from build123d import *

# Parameters (mm, degrees)
F0_R     = 11
F1_DEPTH = 7


# Not quite as in the source:
# - a feature of the source that left no trace in its solid (it failed there, or was rolled back) is left out


with BuildPart() as f1:
    # F0 (on Top) → F1 (new body)
    with BuildSketch(Plane.XY):
        with BuildLine():
            ThreePointArc((10.0491768514, 24.5005127008), (2.4404784534, 18.2483589799), (-7.1242678109, 20.5930010332))
            ThreePointArc((-7.1242678109, 20.5930010332), (-12.6262898219, 5.3096518199), (-26.2426548303, -3.54741391))
            ThreePointArc((-26.2426548303, -3.54741391), (-17.732134245, -6.3123707797), (-14.0924093757, -14.4871093077))
            ThreePointArc((-14.0924093757, -14.4871093077), (-14.1373809935, -15.4807657603), (-14.2719281295, -16.4662974242))
            ThreePointArc((-14.2719281295, -16.4662974242), (1.7148515496, -13.5895136513), (16.1934779789, -20.9530987908))
            ThreePointArc((16.1934779789, -20.9530987908), (14.5833032273, -11.237695828), (21.3961959404, -4.126703609))
            ThreePointArc((21.3961959404, -4.126703609), (10.9114382722, 8.2798618313), (10.0491768514, 24.5005127008))
        make_face()
        Circle(F0_R, mode=Mode.SUBTRACT)
        with BuildLine():
            ThreePointArc((10.0491768514, 24.5005127008), (10.7596687999, 26.6874026373), (11, 28.9742186153))
            ThreePointArc((11, 28.9742186153), (-4.6169824604, 38.9583797198), (-7.1242678109, 20.5930010332))
            ThreePointArc((-7.1242678109, 20.5930010332), (2.4404784534, 18.2483589799), (10.0491768514, 24.5005127008))
        make_face()
        with BuildLine():
            ThreePointArc((-14.0924093757, -14.4871093077), (-17.732134245, -6.3123707797), (-26.2426548303, -3.54741391))
            ThreePointArc((-26.2426548303, -3.54741391), (-33.1610370706, -21.9635554634), (-14.2719281295, -16.4662974242))
            ThreePointArc((-14.2719281295, -16.4662974242), (-14.1373809935, -15.4807657603), (-14.0924093757, -14.4871093077))
        make_face()
        with BuildLine():
            ThreePointArc((36.0924093757, -14.4871093077), (31.4304552974, -5.4966046559), (21.3961959404, -4.126703609))
            ThreePointArc((21.3961959404, -4.126703609), (14.5833032273, -11.237695828), (16.1934779789, -20.9530987908))
            ThreePointArc((16.1934779789, -20.9530987908), (28.4918030448, -24.9486638137), (36.0924093757, -14.4871093077))
        make_face()
    extrude(amount=F1_DEPTH)


solid = f1.part
Geometry check sheet. Reference: the model listing, model coordinates, mm. Coordinates: 2 decimals unless noted, no trailing zeros. Order: outer loops, then holes, each group sorted by start corner. A loop starts at its lowest first (then second) coordinate and runs counter-clockwise, first axis right, second up. Notation, with made-up numbers: (27, 20) -> (47, 20) arc R22 ccw to (47, 26) -> close; hole circle Ø5 at (-40, 3). An arc over 180 degrees is marked (long way). Use a Markdown table: item, result. Add a question column.
1. Cross-section at A-A (y = -18). Enter the section's corners in (x, z), and give its area (3 significant figures).
2. Cross-section at B-B (z = 2.75). Enter the section's corners in (x, y), and give its area (3 significant figures).
3. Go/stop test with flat-tipped pins: pin 1 Ø3 at (x, z) = (18, 5) entering from -Y; pin 2 Ø1 at (y, z) = (1, 3.5) entering from +X; pin 3 Ø2 at (y, z) = (-12.5, 5.5) entering from -X. Record where each tip stops, or that it passes through.
4. Cross-section at D-D (x = -27.5). Enter the section's corners in (y, z).
5. Mould release check, pull along Y, two halves, no side actions. Record for faces 1 (the face through (-9, 8, 0)), 2 (the face through (-12.483, 5.492, 3.451)), 3 (the face through (1.486, -13.557, 3.451)): pulls with the +Y half, pulls with the -Y half, needs draft (parallel to the pull), parting line crosses it, or undercut.
6. Cross-section at C-C (x = 0). Enter the section's corners in (y, z).
7. Material ranges on L1, parallel to Y at x = -0.5, z = 1; L2, parallel to Y at x = 6, z = 4.75; L3, parallel to Y at x = 28, z = 0.5, recorded low to high.
Filled sheet:
| question | item | result |
|---|---|---|
| 1 | outline | (-35.52, 0) -> (-14.67, 0) -> (-14.67, 7) -> (-35.52, 7) -> close; (12.72, 0) -> (35.52, 0) -> (35.52, 7) -> (12.72, 7) -> close |
| 1 | area | 305 mm2 |
| 2 | outline | (-26.24, -3.55) arc R11 ccw (long way) to (-14.27, -16.47) arc R25.49 cw to (16.19, -20.95) arc R11 ccw (long way) to (21.4, -4.13) arc R25.49 cw to (10.05, 24.5) arc R11 ccw (long way) to (-7.12, 20.59) arc R25.49 cw to start; hole circle Ø22 at (0, 0) |
| 2 | area | 1,690 mm2 |
| 3 | pin 1 | y = -23.96 |
| 3 | pin 2 | x = 15.77 |
| 3 | pin 3 | x = -36.05 |
| 4 | outline | (-25.22, 0) -> (-3.75, 0) -> (-3.75, 7) -> (-25.22, 7) -> close |
| 5 | face 1 | needs draft |
| 5 | face 2 | undercut |
| 5 | face 3 | pulls with the -Y half |
| 6 | outline | (-13.4, 0) -> (-11, 0) -> (-11, 7) -> (-13.4, 7) -> close; (11, 0) -> (39.97, 0) -> (39.97, 7) -> (11, 7) -> close |
| 7 | L1 | -13.36 to -10.99, 10.99 to 39.96 |
| 7 | L2 | -14.61 to -9.22, 9.22 to 38.19 |
| 7 | L3 | -25.1 to -3.88 |
